Autodesk Inventor part; units mm, degrees
ref_plane "YZ Plane" through (0, 0, 0) normal (1, 0, 0) x (0, 1, 0)
ref_plane "XZ Plane" through (0, 0, 0) normal (0, 1, 0) x (-1, 0, 0)
ref_plane "XY Plane" through (0, 0, 0) normal (0, 0, 1) x (1, 0, 0)
sketch "Эскиз1" plane through (0, 0, 0) normal (0, 0, 1) x (1, 0, 0)
  line L0 (12, 4) -> (40, 4) construction
  line L1 (0, 0) -> (52, 0) construction
  line L2 (-67.6811, -0.2343) -> (32.3189, -0.2343)
  line L3 (132.3189, 9.7657) -> (132.3189, 23.0512)
  line L4 (-77.6811, 26.4691) -> (-77.6811, 9.7657)
  line L5 (-77.6811, 26.4691) -> (-87.8723, 54.4691)
  line L6 (132.3189, 23.0512) -> (142.51, 51.0512)
  arc A0 (142.51, 51.0512) -> (146.8898, 221.5537) centre (23.3362, 139.42) ccw
  arc A1 (-90.1063, 221.3637) -> (-87.8723, 54.4691) centre (23.3362, 139.42) ccw
  arc A2 (-69.8234, 209.8708) -> (128.2861, 211.2859) centre (29.5436, 166.8699) ccw
  line L7 (-77.1442, 224.2501) -> (-74.1451, 222.5843)
  line L8 (133.7794, 224.7999) -> (132.6234, 224.1703)
  line L9 (-27.6811, 26.8699) -> (82.3189, 26.8699)
  line L10 (32.3189, -0.2343) -> (122.3189, -0.2343)
  line L11 (-37.6811, 36.8699) -> (-37.6811, 63.541)
  line L12 (92.3189, 36.8699) -> (92.3189, 60.779)
  arc A3 (-37.6811, 63.541) -> (92.3189, 60.779) centre (29.5436, 166.8699) ccw
  arc A4 (-37.6811, 36.8699) -> (-27.6811, 26.8699) centre (-27.6811, 36.8699) ccw
  arc A5 (82.3189, 26.8699) -> (92.3189, 36.8699) centre (82.3189, 36.8699) ccw
  arc A6 (-69.8234, 209.8708) -> (-74.1451, 222.5843) centre (-79.0009, 213.8423) ccw
  arc A7 (-77.1442, 224.2501) -> (-90.1063, 221.3637) centre (-82, 215.5082) ccw
  arc A8 (132.6234, 224.1703) -> (128.2861, 211.2859) centre (137.4059, 215.3881) ccw
  arc A9 (146.8898, 221.5537) -> (133.7794, 224.7999) centre (138.562, 216.0177) ccw
  circle A10 centre (5, 17) radius 1.6
  circle A11 centre (5, 10) radius 1.6
  circle A12 centre (47, 10) radius 1.6
  circle A13 centre (47, 17) radius 1.6
  arc A14 (-77.6811, 9.7657) -> (-67.6811, -0.2343) centre (-67.6811, 9.7657) ccw
  arc A15 (122.3189, -0.2343) -> (132.3189, 9.7657) centre (122.3189, 9.7657) ccw
  point P0 (-77.6811, -0.2343)
  point P1 (132.3189, -0.2343)
  point P2 (141.7652, 229.1487)
  point P3 (-65.8946, 218.0014)
  point P4 (26, 0)
  point P5 (77.3189, -0.2343)
  point P6 (-77.6811, 18.1174)
  point P7 (-37.6811, 50.2054)
  point P8 (132.3189, 16.4085)
  point P9 (92.3189, 48.8244)
  dimension "d21" = 167.1042
  dimension "d22" = 10
  dimension "d23" = 10
  dimension "d28" = 100
  dimension "d29" = 15
  dimension "d32" = 140
  dimension "d33" = 10
  dimension "d43" = 100
  dimension "d44" = 40
  dimension "d45" = 40
  dimension "d46" = 28
  dimension "d47" = 28
  dimension "d48" = 20
  dimension "d49" = 20
extrude "Выдавливание1" add sketch "Эскиз1" along normal blind 4
sketch "Эскиз2" plane through (0, 0, 4) normal (0, 0, 1) x (1, 0, 0)
  arc A0 (-77.1442, 224.2501) -> (-90.1063, 221.3637) centre (-82, 215.5082) ccw construction
  line L0 (-37.6811, 36.8699) -> (-37.6811, 63.541) construction
  arc A1 (-77.1442, 224.2501) -> (-37.6811, 50.2054) centre (34.7868, 158.1332) ccw construction
  circle A2 centre (-91.995, 129.3866) radius 2.1
  circle A3 centre (-72.2713, 84.3866) radius 2.1
  circle A4 centre (-94.1931, 174.3866) radius 2.1
  line L1 (-67.6811, -0.2343) -> (122.3189, -0.2343) construction
  circle A5 centre (5, 10) radius 1.6 construction
  circle A6 centre (47, 10) radius 1.6 construction
  line L2 (5, 10) -> (47, 10) construction
  line L3 (26, 10) -> (26, 211.5399) construction
  line L4 (92.3189, 60.779) -> (92.3189, 36.8699)
  arc A7 (132.6234, 224.1703) -> (128.2861, 211.2859) centre (137.4059, 215.3881) ccw
  arc A8 (92.3189, 48.8244) -> (132.6234, 224.1703) centre (21.0087, 157.5206) ccw construction
  line L5 (-72.2713, 84.3866) -> (128.4862, 84.3866) construction
  circle A9 centre (128.4862, 84.3866) radius 2.1
  line L6 (-91.995, 129.3866) -> (161.5686, 129.3866) construction
  circle A10 centre (147.9279, 129.3866) radius 2.1
  line L7 (-94.1931, 174.3866) -> (161.5686, 174.3866) construction
  circle A11 centre (149.91, 174.3866) radius 2.1
  point P0 (0, 0)
  dimension "d35" = 4.2
  dimension "d36" = 4.2
  dimension "d37" = 45
  dimension "d38" = 4.2
  dimension "d39" = 45
  dimension "d50" = 130
  dimension "d51" = 130
  dimension "d52" = 4.2
  dimension "d53" = 4.2
  dimension "d54" = 4.2
extrude "Выдавливание2" cut sketch "Эскиз2" against normal blind 4
properties part number "фанера_ухо"
Geometry: final body of the model. Coordinates: model frame, mm. A direction names the side the tool comes from. Give positions to 0.01 mm unless a question says otherwise; leave off trailing zeros. Order: outer loops, then holes, each group sorted by start corner. A loop starts at its lowest first (then second) coordinate and runs counter-clockwise, first axis right, second up. Notation, with made-up numbers: (25, 71.5) -> (69, 71.5) arc R5 ccw to (69, 75.5) -> close; hole circle Ø2 at (82, 43.5). An arc over 180 degrees is marked (long way). Write each question's results on one line, items separated by ' | '. Start each with the question number.
1) Section A-A (y = 198). Return loops of the section in (x, z).
2) Set-up query: faces 4 (the cylindrical face through (89.47, 29.88, 1.97)), 5 (the cylindrical face through (-116.57, 136.3, 1.97)). Return all of +Z, -Z, +X, -X, +Y, -Y with unobstructed straight access to the full face (end or side cutting, diameter ignored); none if empty.
3) Section B-B (x = 66). Return loops of the section in (y, z), then the cut area to 3 significant figures.
4) Draft query along X for faces 1 (the flat face through (137.343, 36.855, 1.972)), 2 (the cylindrical face through (-74.674, 2.617, 1.972)), 3 (the cylindrical face through (-34.67, 29.72, 1.97)). Return one class per face: pulls with the +X half, pulls with the -X half, needs draft (parallel to the pull), parting line crosses it, or undercut.
5) Line query: line 1 (Y direction, x = 5, z = 1.95); line 2 (X direction, y = 13.5, z = 2); line 3 (X direction, y = 200, z = 3.2). Output: solid intervals per line, ascending. Write a range as from..to.
6) First-contact query: pin 1 (5.5 mm diameter, centred on x = 149.91, y = 174.39, fed in from +Z); pin 2 (2 mm diameter, centred on y = 15, z = 1, fed in from +X); pin 3 (1.2 mm diameter, centred on y = 21.5, z = 2, fed in from -X); pin 4 (1.2 mm diameter, centred on y = 53, z = 3, fed in from +X). Flat tips, straight axial feed; report the tip coordinate or a pass-through.
7) Section D-D (x = 114.5). Return loops of the section in (y, z), then the cut area to 3 significant figures.
8) Section C-C (z = 1.6). Count the separate pieces of the cut face and the enclosed holes in it, then the cut area to 3 significant figures.
Calculated:
1) outline: (-103.76, 0) -> (-74.16, 0) -> (-74.16, 4) -> (-103.76, 4) -> close; (133.24, 0) -> (159.64, 0) -> (159.64, 4) -> (133.24, 4) -> close
2) face 4: +Z, -Z | face 5: +Z, -Z, -X
3) outline: (-0.23, 0) -> (26.87, 0) -> (26.87, 4) -> (-0.23, 4) -> close; (49.11, 0) -> (64.92, 0) -> (64.92, 4) -> (49.11, 4) -> close | area: 172 mm2
4) face 1: pulls with the +X half | face 2: pulls with the -X half | face 3: undercut
5) line 1: -0.23..8.4, 11.6..15.4, 18.6..26.87, 46.07..61.42 | line 2: -77.68..132.32 | line 3: -102.81..-73.54, 132.62..158.77
6) pin 1: z = 4 | pin 2: x = 132.32 | pin 3: x = -77.68 | pin 4: x = 144.36
7) outline: (-0.23, 0) -> (99.75, 0) -> (99.75, 4) -> (-0.23, 4) -> close | area: 400 mm2
8) separate pieces: 1 | enclosed holes: 11 | area: 24,400 mm2
